from build123d import *

# Parameters (mm, degrees)
SKETCH1_R           = 3.3782
BOSS_EXTRUDE1_DEPTH = 3.175


with BuildPart() as part:
    # Sketch1 → Boss-Extrude1 (new body)
    with BuildSketch(Plane.XY):
        with BuildLine():
            Line((-2.54, 39.37), (2.54, 39.37))
            add(Edge.make_bspline(
                [(2.54, 39.37), (9.095418915, 34.201637521), (9.525, 25.4)],
                knots=[0, 0, 0, 1, 1, 1], degree=2))
            Line((9.525, 25.4), (9.525, 0.833077402))
            Line((9.525, 0.833077402), (13.080713372, -25.725670045))
            Line((13.080713372, -25.725670045), (49.772779476, -31.025635149))
            Line((49.772779476, -31.025635149), (49.772779476, -38.975582805))
            Line((49.772779476, -38.975582805), (10.326960053, -38.975582805))
            Line((10.326960053, -38.975582805), (0, -31.025635149))
            Line((0, -31.025635149), (-9.525, 0))
            Line((-9.525, 0), (-9.525, 25.4))
            add(Edge.make_bspline(
                [(-2.54, 39.37), (-9.095418915, 34.201637521), (-9.525, 25.4)],
                knots=[0, 0, 0, 1, 1, 1], degree=2))
        make_face()
        with Locations((0, 25.4)):
            Circle(SKETCH1_R, mode=Mode.SUBTRACT)
        Circle(SKETCH1_R, mode=Mode.SUBTRACT)
    extrude(amount=BOSS_EXTRUDE1_DEPTH)


solid = part.part
Part model, mm, in its own coordinate system. A direction names the side the tool comes from. Coordinates: 2 decimals unless noted, no trailing zeros. Order: outer loops, then holes, each group sorted by start corner. A loop starts at its lowest first (then second) coordinate and runs counter-clockwise, first axis right, second up. Notation, with made-up numbers: M 2.25,62.5 L 10.25,62.5 A21 cw 10.25,77.5 Z; hole C 78.5,-22.5 d10. An arc over 180 degrees is marked long. Use a Markdown table: item, result.
(1) Probe L1, parallel to X at y = 9, z = 2.6 (3 decimals); L2, parallel to Y at x = 0.5, z = 1.8; L3, parallel to Y at x = 42.5, z = 1.5. List the from-to ranges inside material, lowest first.
A:
| item | result |
|---|---|
| L1 | x = -9.525 to 9.525 |
| L2 | y = -31.41 to -3.34, 3.34 to 22.06, 28.74 to 39.37 |
| L3 | y = -38.98 to -29.98 |
(2) Cut at A-A on x = -1. Write the cut outline in (y, z) (3 decimals).
A:
| item | result |
|---|---|
| outline | M -27.768,0 L -3.227,0 L -3.227,3.175 L -27.768,3.175 Z; M 3.227,0 L 22.173,0 L 22.173,3.175 L 3.227,3.175 Z; M 28.627,0 L 39.37,0 L 39.37,3.175 L 28.627,3.175 Z |
(3) Cut at D-D on x = 18. Write the cut outline in (y, z) (3 decimals).
A:
| item | result |
|---|---|
| outline | M -38.976,0 L -26.436,0 L -26.436,3.175 L -38.976,3.175 Z |
(4) Cut at B-B on z = 1.55. State how many separate pieces and enclosed holes the cut face has, then the cut area to 3 significant figures.
A:
| item | result |
|---|---|
| separate pieces | 1 |
| enclosed holes | 2 |
| area | 1,580 mm^2 |
(5) Flat gauge pin, fed straight in: pin 1 (2 mm diameter, centred on x = -2.5, y = 21.5, fed in from -Z). Where does the tip first touch, or does it go through?
A:
| item | result |
|---|---|
| pin 1 | stops at z = 0 |
(6) Cut at C-C on y = -20. Write the cut outline in (x, z) (3 decimals), then the cut area to 3 significant figures.
A:
| item | result |
|---|---|
| outline | M -3.385,0 L 12.314,0 L 12.314,3.175 L -3.385,3.175 Z |
| area | 49.8 mm^2 |
(7) Pull direction Y, two halves, no side cores. Call faces 1 (the flat face through (30, -38.976, 2)), 2 (the flat face through (49.773, -35, 2)), 3 (the cylindrical face through (-0.73, 22.1, 1.57)): released by +Y, released by -Y, zero draft, split by the parting line, or undercut.
A:
| item | result |
|---|---|
| face 1 | released by -Y |
| face 2 | zero draft |
| face 3 | undercut |
(8) Tool access for faces 4 (the cylindrical face through (-2.681, -2.056, 1.565)), 5 (the flat face through (9.525, 13, 2)): list every direction of +Z, -Z, +X, -X, +Y, -Y with a clear straight run to the whole face (end or side of a thin tool).
A:
| item | result |
|---|---|
| face 4 | +Z, -Z |
| face 5 | +Z, -Z, +X, +Y |
